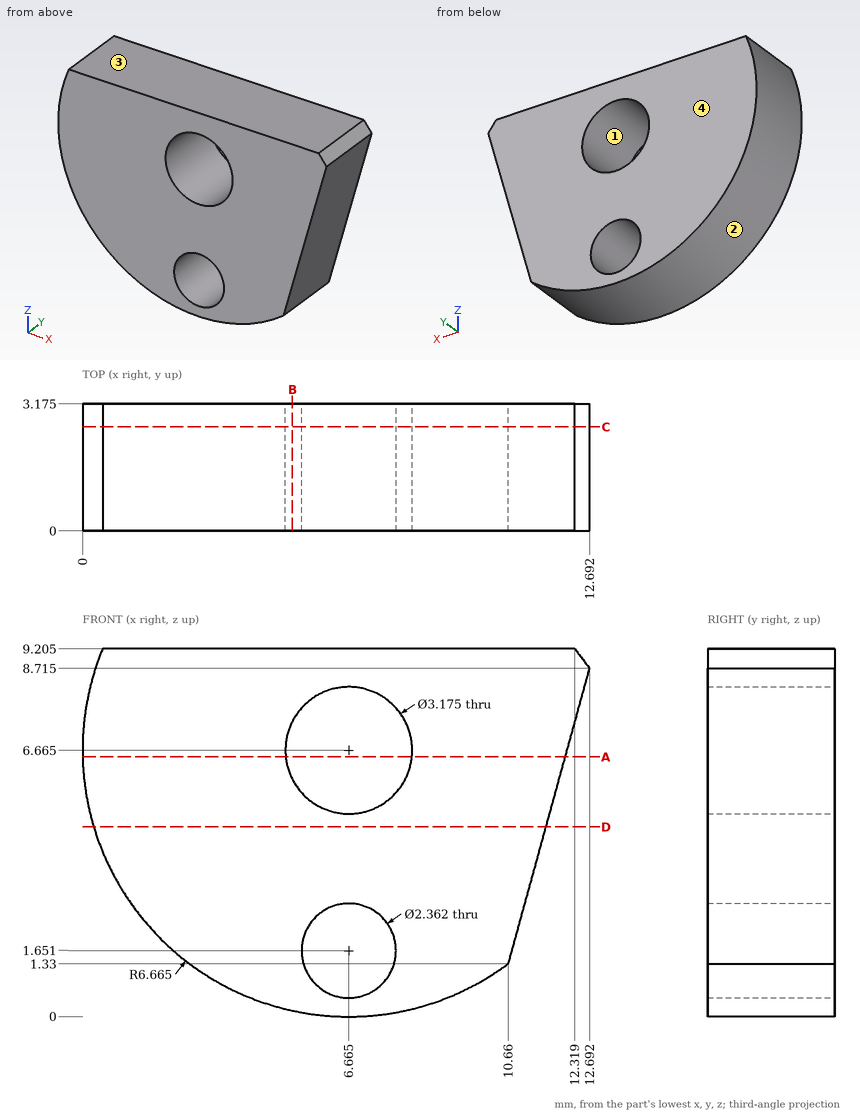
Answer from the drawing. Dimensions are ordinates in mm from the lowest x, y and z of the part. Coordinates: 2 decimals unless noted, no trailing zeros. Loops run counter-clockwise (first coordinate to the right, second up) from the corner with the lowest first, then second, coordinate; pieces in that order, holes last. Notation, with made-up numbers: (83.5, 29) -> (115.5, 29) arc R29 cw to (115.5, 57) -> close; hole circle Ø1 at (51, 39). An arc over 180 degrees is marked (long way). Answer as CSV lines item,"result".
Q1. The part is cut by section B-B on x = 5.25. Write down the section's boundary in (y, z) (1 decimal).
Findings:
outline,"(0, 0.2) -> (3.2, 0.2) -> (3.2, 5.9) -> (0, 5.9) -> close; (0, 7.4) -> (3.2, 7.4) -> (3.2, 9.2) -> (0, 9.2) -> close"
Q2. The part is cut by section A-A on z = 6.5. Write down the section's boundary in (x, y) (1 decimal).
Findings:
outline,"(0, 0) -> (5.1, 0) -> (5.1, 3.2) -> (0, 3.2) -> close; (8.2, 0) -> (12.1, 0) -> (12.1, 3.2) -> (8.2, 3.2) -> close"
Q3. This flat-tipped pin is pushed along its axis until it touches: pin 1 (3 mm diameter, centred on x = 6.66, z = 6.66, fed in from +Y). Where does it stop, or does it pass through?
Findings:
pin 1,"passes through"
Q4. Find the intervals of material crossed by probe 1 along Z at (x, y) = (7, 2.15) (1 decimal); probe 2 along Z at (x, y) = (6, 2.8) (1 decimal); probe 3 along X at (y, z) = (2.95, 7), in increasing order.
Findings:
probe 1,"z = 0 to 0.5, 2.8 to 5.1, 8.2 to 9.2"
probe 2,"z = 0 to 0.7, 2.6 to 5.2, 8.1 to 9.2"
probe 3,"x = 0.01 to 5.11, 8.22 to 12.22"
Q5. The part is cut by section D-D on z = 4.75. Write down the section's boundary in (x, y) (1 decimal).
Findings:
outline,"(0.3, 0) -> (11.6, 0) -> (11.6, 3.2) -> (0.3, 3.2) -> close"
Q6. The part is cut by section C-C on y = 2.6. Write down the section's boundary in (x, z) (1 decimal).
Findings:
outline,"(0.5, 9.2) arc R6.7 ccw to (10.7, 1.3) -> (12.7, 8.7) -> (12.3, 9.2) -> close; hole circle Ø3.2 at (6.7, 6.7); hole circle Ø2.4 at (6.7, 1.7)"
Q7. For a pull along Z with two mould halves and no side action, classify the marked faces 1, 2, 3 and 4 as +Z half, -Z half, draft (parallel to the pull), parting line (faces both ways), or undercut.
Findings:
face 1,"undercut"
face 2,"parting line"
face 3,"+Z half"
face 4,"draft"
